from build123d import *

# Parameters (mm, degrees)
F0_R     = 12.5
F1_DEPTH = 5
F2_W     = 10.5
F2_H     = 5.25
F3_DEPTH = 4


with BuildPart() as f1:
    # F0 (on Top) → F1 (new body)
    with BuildSketch(Plane.XY):
        Circle(F0_R)
    extrude(amount=F1_DEPTH)


with BuildPart() as f3:
    # F2 (on face) → F3 (new body)
    with BuildSketch(Plane.XY.offset(5)):
        with Locations((0, 5.625)):
            Rectangle(F2_W, F2_H)
        with Locations((0, -5.625)):
            Rectangle(F2_W, F2_H)
    extrude(amount=-F3_DEPTH)


with BuildPart() as f1_1:
    add(f1.part)

    # F4: cut F3
    add(f3.part, mode=Mode.SUBTRACT)


solid = f1_1.part
For this review, take the finished solid that the model builds, in its own axes (mm). A direction names the side the tool comes from. Give positions to 0.01 mm unless a question says otherwise; leave off trailing zeros. Order: outer loops, then holes, each group sorted by start corner. A loop starts at its lowest first (then second) coordinate and runs counter-clockwise, first axis right, second up. Notation, with made-up numbers: (-37, 25.5) -> (-31, 25.5) arc R20 cw to (-31, 43.5) -> close; hole circle Ø9 at (74, 43.25). An arc over 180 degrees is marked (long way). Write item = value, one per line.
1) We need section B-B, the plane x = 0. Give the boundary of the cut face in (y, z).
Findings:
outline = (-12.5, 0) -> (12.5, 0) -> (12.5, 5) -> (8.25, 5) -> (8.25, 1) -> (3, 1) -> (3, 5) -> (-3, 5) -> (-3, 1) -> (-8.25, 1) -> (-8.25, 5) -> (-12.5, 5) -> close
2) To check wall thickness, follow L1, parallel to Y at x = -5, z = 4.3; L2, parallel to Z at x = 3, y = -4.25; L3, parallel to Y at x = 3.5, z = 2.7. State the ranges of each line that lie inside material, in increasing order. Write a range as from..to.
Findings:
L1 = -11.46..-8.25, -3..3, 8.25..11.46
L2 = 0..1
L3 = -12..-8.25, -3..3, 8.25..12
3) We need section D-D, the plane x = 6.25. Give the boundary of the cut face in (y, z), and give its area (3 significant figures).
Findings:
outline = (-10.83, 0) -> (10.83, 0) -> (10.83, 5) -> (-10.83, 5) -> close
area = 108 mm^2
4) For faces 1 (the face through (0, -6, 1)), 2 (the face through (0, 0, 5)), list the 3-axis set-ups (+Z, -Z, +X, -X, +Y, -Y) from which the entire face can be reached by the end or side of a thin tool; tool diameter is ignored.
Findings:
face_1 = +Z
face_2 = +Z, +X, -X, +Y, -Y
5) Draft analysis for pull direction X (two halves, no side actions). For faces 3 (the face through (5.25, -6, 3)), 4 (the face through (0, 0, 0)), 5 (the face through (-5.25, 6, 3)), 6 (the face through (11.923, 3.755, 2.465)), state which applies: pulls with the +X half, pulls with the -X half, needs draft (parallel to the pull), parting line crosses it, or undercut.
Findings:
face_3 = undercut
face_4 = needs draft
face_5 = undercut
face_6 = parting line crosses it
6) We need section C-C, the plane y = -3.5. Give the boundary of the cut face in (x, z).
Findings:
outline = (-12, 0) -> (12, 0) -> (12, 5) -> (5.25, 5) -> (5.25, 1) -> (-5.25, 1) -> (-5.25, 5) -> (-12, 5) -> close
7) We need section A-A, the plane z = 3.65. Give the boundary of the cut face in (x, y).
Findings:
outline = circle Ø25 at (0, 0); hole (-5.25, -8.25) -> (5.25, -8.25) -> (5.25, -3) -> (-5.25, -3) -> close; hole (-5.25, 3) -> (5.25, 3) -> (5.25, 8.25) -> (-5.25, 8.25) -> close
8) Insertion check: pin 1 (1.2 mm diameter, centred on y = 4.5, z = 3, fed in from +X); pin 2 (3 mm diameter, centred on y = -9.5, z = 1.5, fed in from +X); pin 3 (3 mm diameter, centred on y = 7.5, z = 3.5, fed in from +X). Each pin has a flat end and moves straight along its axis. Give the tip position at first contact, or say it passes through.
Findings:
pin_1 = 11.88
pin_2 = 9.6
pin_3 = 10.97
